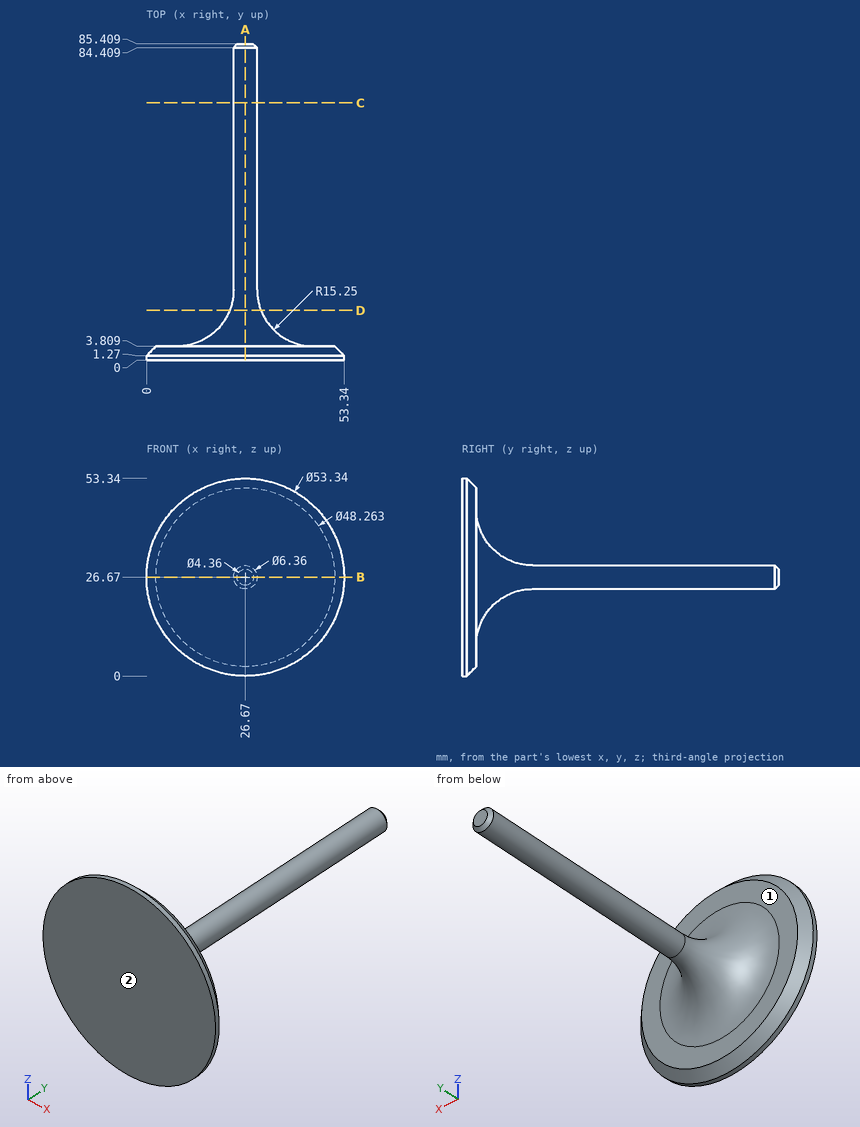
The figure shows three views and two pictorial views of one solid part (mm, origin at its lowest corner). Answer the questions. A direction names the side the tool comes from. Coordinates: 2 decimals unless noted, no trailing zeros. Loops run counter-clockwise (first coordinate to the right, second up) from the corner with the lowest first, then second, coordinate; pieces in that order, holes last. Notation, with made-up numbers: (-1, -11.5) - (27, -11.5) arc R18 cw to (27, 7.5) - close; hole circle Ø5 at (-25, -5.5). An arc over 180 degrees is marked (long way). Answer in a Markdown table with one row per item.
Q1. Given P1, Ø3, axis at y = 53.5, z = 25, coming from the -X side (1 decimal); P2, Ø4, axis at x = 22.5, y = 30, coming from the +Z side (1 decimal); P3, Ø6, axis at y = 52, z = 17.5, coming from the +X side, each flat-ended and moving along its own axis, determine where each tip first touches the part or whether it passes through.
Here are the results:
| item | result |
|---|---|
| P1 | stops at x = 23.5 |
| P2 | stops at z = 29 |
| P3 | passes through |
Q2. For the marked faces 1 and 2, determine the directions among +Z, -Z, +X, -X, +Y, -Y from which every point of the face is accessible in a straight line to the end or side of a thin tool.
Here are the results:
| item | result |
|---|---|
| face 1 | +Y |
| face 2 | +Z, -Z, +X, -X, -Y |
Q3. Find section C-C on y = 69.5. Write down the section's boundary in (x, z).
Here are the results:
| item | result |
|---|---|
| outline | circle Ø6.36 at (26.67, 26.67) |
Q4. Find section A-A on x = 26.67. Write down the section's boundary in (y, z).
Here are the results:
| item | result |
|---|---|
| outline | (0, 0) - (1.27, 0) - (3.81, 2.54) - (3.81, 8.24) arc R15.25 cw to (19.06, 23.49) - (84.41, 23.49) - (85.41, 24.49) - (85.41, 28.85) - (84.41, 29.85) - (19.06, 29.85) arc R15.25 cw to (3.81, 45.1) - (3.81, 50.8) - (1.27, 53.34) - (0, 53.34) - close |
Q5. Straight lines are drawn through the part: line 1 along Y through (x, z) = (19, 49); line 2 along Z through (x, y) = (28, 38); line 3 along Y through (x, z) = (32, 33). For each, find the intervals that lie inside material, in ascending order. Write a range as [from, to].
Here are the results:
| item | result |
|---|---|
| line 1 | y = [0, 3.81] |
| line 2 | z = [23.78, 29.56] |
| line 3 | y = [0, 7.68] |
Q6. Find section D-D on y = 13.5. Write down the section's boundary in (x, z), plus the area to 3 significant figures.
Here are the results:
| item | result |
|---|---|
| outline | circle Ø8.46 at (26.67, 26.67) |
| area | 56.2 mm^2 |
Q7. Find section B-B on z = 26.67. Write down the section's boundary in (x, y).
Here are the results:
| item | result |
|---|---|
| outline | (0, 0) - (53.34, 0) - (53.34, 1.27) - (50.8, 3.81) - (45.1, 3.81) arc R15.25 cw to (29.85, 19.06) - (29.85, 84.41) - (28.85, 85.41) - (24.49, 85.41) - (23.49, 84.41) - (23.49, 19.06) arc R15.25 cw to (8.24, 3.81) - (2.54, 3.81) - (0, 1.27) - close |
